from build123d import *

# Parameters (mm, degrees)
BOSS_EXTRUDE2_DEPTH = 4
CUT_EXTRUDE1_DEPTH  = 10
SKETCH3_R           = 7.5
SKETCH3_R_2         = 10
CUT_EXTRUDE2_DEPTH  = 10


with BuildPart() as part:
    # Sketch1 → Boss-Extrude2 (new body)
    with BuildSketch(Plane.XY):
        Polygon((-75, -201), (-10, -201), (-10, -205), (10, -205), (10, -201), (75, -201), (75, -205), (91, -205), (91, -191), (95, -191), (95, -171), (91, -171), (91, -81), (95, -81), (95, -61), (91, -61), (91, 61), (95, 61), (95, 81), (91, 81), (91, 171), (95, 171), (95, 191), (91, 191), (91, 205), (75, 205), (75, 201), (10, 201), (10, 205), (-10, 205), (-10, 201), (-75, 201), (-75, 205), (-91, 205), (-91, 191), (-95, 191), (-95, 171), (-91, 171), (-91, 81), (-95, 81), (-95, 61), (-91, 61), (-91, -61), (-95, -61), (-95, -81), (-91, -81), (-91, -171), (-95, -171), (-95, -191), (-91, -191), (-91, -205), (-75, -205), align=None)
        with BuildLine():
            Line((-17.949055326, 171.697819396), (17.949055326, 171.697819396))
            ThreePointArc((17.949055326, 171.697819396), (32.09119095, 165.83995502), (37.949055326, 151.697819396))
            Line((37.949055326, 151.697819396), (37.949055326, 56.741742537))
            ThreePointArc((37.949055326, 56.741742537), (32.09119095, 42.599606914), (17.949055326, 36.741742537))
            Line((17.949055326, 36.741742537), (-17.949055326, 36.741742537))
            ThreePointArc((-17.949055326, 36.741742537), (-32.09119095, 42.599606914), (-37.949055326, 56.741742537))
            Line((-37.949055326, 56.741742537), (-37.949055326, 151.697819396))
            ThreePointArc((-37.949055326, 151.697819396), (-32.09119095, 165.83995502), (-17.949055326, 171.697819396))
        make_face(mode=Mode.SUBTRACT)
        with BuildLine():
            Line((-17.949055326, -166.180135652), (17.949055326, -166.180135652))
            ThreePointArc((17.949055326, -166.180135652), (32.09119095, -160.322271276), (37.949055326, -146.180135652))
            Line((37.949055326, -146.180135652), (37.949055326, -60))
            ThreePointArc((37.949055326, -60), (32.09119095, -45.857864376), (17.949055326, -40))
            Line((17.949055326, -40), (-17.949055326, -40))
            ThreePointArc((-17.949055326, -40), (-32.09119095, -45.857864376), (-37.949055326, -60))
            Line((-37.949055326, -60), (-37.949055326, -146.180135652))
            ThreePointArc((-37.949055326, -146.180135652), (-32.09119095, -160.322271276), (-17.949055326, -166.180135652))
        make_face(mode=Mode.SUBTRACT)
    extrude(amount=BOSS_EXTRUDE2_DEPTH)

    # Sketch2 → Cut-Extrude1 (cut)
    with BuildSketch(Plane.XY.offset(4)):
        with BuildLine():
            Line((0, -40), (58.886613453, -40))
            ThreePointArc((58.886613453, -40), (69.49321517, -44.393398282), (73.886613453, -55))
            Line((73.886613453, -55), (73.886613453, -96.0450181))
            ThreePointArc((73.886613453, -96.0450181), (69.49321517, -106.651619817), (58.886613453, -111.0450181))
            Line((58.886613453, -111.0450181), (0, -111.0450181))
            Line((0, -111.0450181), (0, -40))
        make_face()
    extrude(amount=-CUT_EXTRUDE1_DEPTH, mode=Mode.SUBTRACT)

    # Sketch3 → Cut-Extrude2 (cut)
    with BuildSketch(Plane.XY.offset(4)):
        with Locations((-65.497286905, 22.916669932)):
            Circle(SKETCH3_R)
        with Locations((-65.497286905, -6.583495202)):
            Circle(SKETCH3_R_2)
    extrude(amount=-CUT_EXTRUDE2_DEPTH, mode=Mode.SUBTRACT)


solid = part.part
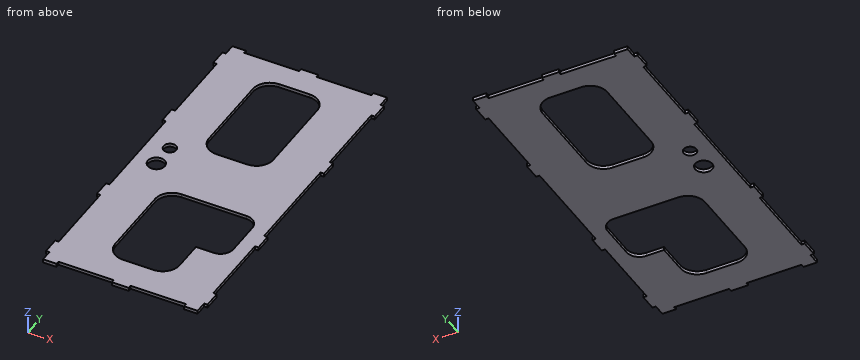
Build history of the part. All positions in model axes, mm. Give positions to 0.01 mm unless a question says otherwise; leave off trailing zeros. Order: outer loops, then holes, each group sorted by start corner. A loop starts at its lowest first (then second) coordinate and runs counter-clockwise, first axis right, second up. Notation, with made-up numbers: M -32.75,39.5 L 18.25,39.5 A28 ccw 18.25,58.5 Z; hole C 89,3 d8. An arc over 180 degrees is marked long. Use one line per item in the form item = value.
1) Drop flat-ended pins along their axis: pin 1 (12 mm diameter, centred on x = -65.5, y = -6.58, fed in from +Z); pin 2 (1.5 mm diameter, centred on y = -114, z = 0.5, fed in from +X); pin 3 (1.2 mm diameter, centred on y = 203.5, z = 3, fed in from -X); pin 4 (2 mm diameter, centred on x = 56, z = 2, fed in from +Y). Give the stop position or say it passes through.
Calculated:
pin_1 = through
pin_2 = 91
pin_3 = -91
pin_4 = 201
2) Probe probe 1 along Y at (x, z) = (11, 2.6); probe 2 along X at (y, z) = (139, 1.75); probe 3 along Y at (x, z) = (-68, 3.7). List the from-to ranges inside material, lowest first.
Calculated:
probe_1 = -201 to -166.18, -40 to 36.74, 171.7 to 201
probe_2 = -91 to -37.95, 37.95 to 91
probe_3 = -201 to -16.27, 3.1 to 15.85, 29.99 to 201
3) Saw through at B-B (y = 132.5). Give the cut face in (x, z), plus the area to 3 significant figures.
Calculated:
outline = M -91,0 L -37.95,0 L -37.95,4 L -91,4 Z; M 37.95,0 L 91,0 L 91,4 L 37.95,4 Z
area = 424 mm2
4) Saw through at A-A (y = -90). Give the cut face in (x, z), plus the area to 3 significant figures.
Calculated:
outline = M -91,0 L -37.95,0 L -37.95,4 L -91,4 Z; M 73.89,0 L 91,0 L 91,4 L 73.89,4 Z
area = 281 mm2
5) Saw through at C-C (z = 1.5). State how many separate pieces and enclosed holes the cut face has, plus the area to 3 significant figures.
Calculated:
separate_pieces = 1
enclosed_holes = 4
area = 52,100 mm2
